Verification items for this drawing (mm, ordinates from the low corner). Round coordinates to 2 decimals unless told otherwise and drop trailing zeros. Loops run counter-clockwise (first coordinate to the right, second up) from the corner with the lowest first, then second, coordinate; pieces in that order, holes last. Notation, with made-up numbers: (-18.75, -15) - (2.25, -15) arc R28 cw to (2.25, 3) - close; hole circle Ø1 at (29.5, 1.5). An arc over 180 degrees is marked (long way). Answer in a Markdown table with one row per item. Add a question column.
(1) Cross-section at C-C on x = 325. Enter the section's corners in (y, z), then the cut area to 3 significant figures.
(2) Cross-section at A-A on y = 65. Enter the section's corners in (x, z), then the cut area to 3 significant figures.
(3) Cross-section at B-B on x = 65. Enter the section's corners in (y, z), then the cut area to 3 significant figures.
(4) Thickness scan on line 1 along Y through (x, z) = (65, 3.4); line 2 along X through (y, z) = (325, 1.2); line 3 along Y through (x, z) = (327, 3.15). Record the ranges inside material, lowest first.
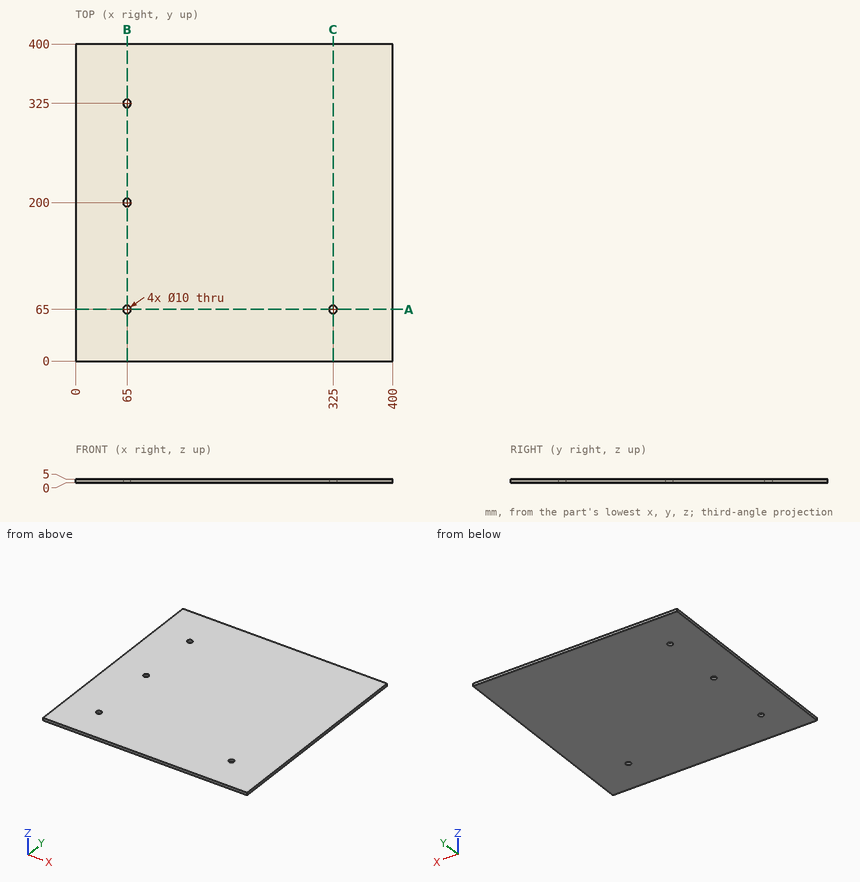
Answers:
| question | item | result |
|---|---|---|
| 1 | outline | (0, 0) - (60, 0) - (60, 5) - (0, 5) - close; (70, 0) - (400, 0) - (400, 5) - (70, 5) - close |
| 1 | area | 1,950 mm^2 |
| 2 | outline | (0, 0) - (60, 0) - (60, 5) - (0, 5) - close; (70, 0) - (320, 0) - (320, 5) - (70, 5) - close; (330, 0) - (400, 0) - (400, 5) - (330, 5) - close |
| 2 | area | 1,900 mm^2 |
| 3 | outline | (0, 0) - (60, 0) - (60, 5) - (0, 5) - close; (70, 0) - (195, 0) - (195, 5) - (70, 5) - close; (205, 0) - (320, 0) - (320, 5) - (205, 5) - close; (330, 0) - (400, 0) - (400, 5) - (330, 5) - close |
| 3 | area | 1,850 mm^2 |
| 4 | line 1 | y = 0 to 60, 70 to 195, 205 to 320, 330 to 400 |
| 4 | line 2 | x = 0 to 60, 70 to 400 |
| 4 | line 3 | y = 0 to 60.42, 69.58 to 400 |
